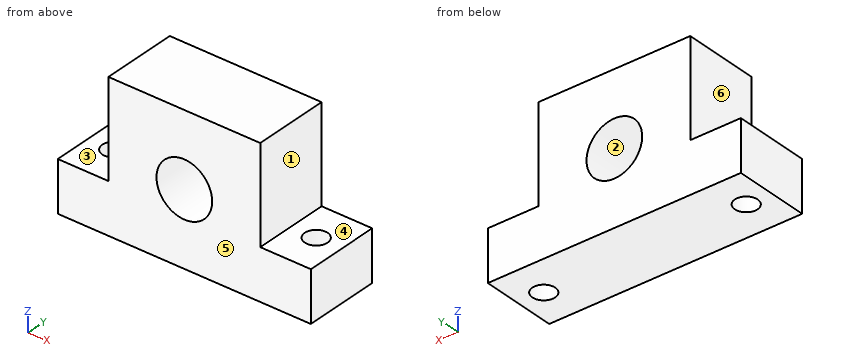
```python
from build123d import *

# Parameters (mm, degrees)
BOSS_EXTRUDE1_DEPTH  = 58
SKETCH3_R            = 11
CUT_EXTRUDE1_DEPTH   = 77.774006375
SKETCH4_W            = 20
SKETCH4_H            = 30
CUT_EXTRUDE2_DEPTH   = 38
M8_CLEARANCE_HOLE1_D = 9


with BuildPart() as part:
    # Sketch1 → Boss-Extrude1 (new body)
    with BuildSketch(Plane(origin=(0, 2.518676762, -29.699029015), x_dir=(1, 0, 0), z_dir=(0, 0, 1))):
        Polygon((-64.126560257, 671.967635092), (-14.126560257, 671.967635092), (35.873439743, 671.967635092), (35.873439743, 701.967635092), (-64.126560257, 701.967635092), align=None)
    extrude(amount=BOSS_EXTRUDE1_DEPTH)

    # Sketch3 → Cut-Extrude1 (cut, through all)
    with BuildSketch(Plane.XZ.offset(-674.486311854)):
        with Locations(Location((-14.126560257, -0.699029015, 0), (0, 0, 270))):
            Circle(SKETCH3_R)
    extrude(amount=-CUT_EXTRUDE1_DEPTH, mode=Mode.SUBTRACT)

    # Sketch4 → Cut-Extrude2 (cut)
    with BuildSketch(Plane.XY.offset(28.300970985)):
        with Locations((-54.126560257, 689.486311854)):
            Rectangle(SKETCH4_W, SKETCH4_H)
        with Locations((25.873439743, 689.486311854)):
            Rectangle(SKETCH4_W, SKETCH4_H)
    extrude(amount=-CUT_EXTRUDE2_DEPTH, mode=Mode.SUBTRACT)

    # M8 Clearance Hole1 (through all)
    with Locations(Plane(origin=(-5.422124321, 631.407959219, -9.699029015), x_dir=(1, 0, 0), z_dir=(0, 0, 1))):
        with Locations((-48.704435936, -458.836111538), (-48.704435936, -493.836111538), (31.295564064, -458.836111538), (31.295564064, -493.836111538), (-48.704435936, 58.078352635), (31.295564064, 58.078352635)):
            Hole(M8_CLEARANCE_HOLE1_D / 2)


solid = part.part
```
Geometry: final body of the model. Coordinates: model frame, mm. Face numbers are marked on the shaded views. A direction names the side the tool comes from. Coordinates: 2 decimals unless noted, no trailing zeros. Order: outer loops, then holes, each group sorted by start corner. A loop starts at its lowest first (then second) coordinate and runs counter-clockwise, first axis right, second up. Notation, with made-up numbers: M 45,62.25 L 90,62.25 A35 ccw 90,95.25 Z; hole C -28,68 d3. An arc over 180 degrees is marked long. Answer in a Markdown table with one row per item. Add a question column.
Q1. Reachability of the marked faces 4, 5 and 6 from +Z, -Z, +X, -X, +Y, -Y: full face, straight path, thin tool, end or side. Return the list, or none.
Q2. Section query B-B on x = 22.5. Return the cut outline in (y, z).
Q3. Section query C-C on y = 684. Return the cut outline in (x, z).
Q4. Section query A-A on z = -8. Return the cut outline in (x, y).
Q5. Line query: L1, parallel to Z at x = -14, y = 689; L2, parallel to Z at x = -45, y = 679.5; L3, parallel to X at y = 687, z = 2. Output: solid intervals per line, ascending.
Q6. Contact query for flat-ended pins moving along their axis: P1, Ø15, axis at y = 691, z = 10.5, coming from the -X side; P2, Ø16, axis at x = 30.5, y = 693.5, coming from the +Z side. Output: stop coordinate, or through.
Q7. Section query D-D on z = -16. Return the cut outline in (x, y).
Q8. Mould query, pull axis Z, two halves, no side actions, for the marked faces 1, 2 and 3. Classes: released by +Z, released by -Z, zero draft, split by the parting line, or undercut.
Completed:
| question | item | result |
|---|---|---|
| 1 | face 4 | +Z, +X, +Y, -Y |
| 1 | face 5 | +Z, -Z, +X, -X, -Y |
| 1 | face 6 | +Z, -X, +Y, -Y |
| 2 | outline | M 674.49,-29.7 L 686.51,-29.7 L 686.51,-9.7 L 674.49,-9.7 Z; M 692.46,-29.7 L 704.49,-29.7 L 704.49,-9.7 L 692.46,-9.7 Z |
| 3 | outline | M -64.13,-29.7 L 35.87,-29.7 L 35.87,-9.7 L 15.87,-9.7 L 15.87,28.3 L -44.13,28.3 L -44.13,-9.7 L -64.13,-9.7 Z; hole C -14.13,-0.7 d22 |
| 4 | outline | M -44.13,674.49 L -22.35,674.49 L -22.35,704.49 L -44.13,704.49 Z; M -5.9,674.49 L 15.87,674.49 L 15.87,704.49 L -5.9,704.49 Z |
| 5 | L1 | z = -29.7 to -11.7, 10.3 to 28.3 |
| 5 | L2 | z = -29.7 to -9.7 |
| 5 | L3 | x = -44.13 to -24.79, -3.46 to 15.87 |
| 6 | P1 | stops at x = -44.13 |
| 6 | P2 | stops at z = -9.7 |
| 7 | outline | M -64.13,674.49 L 35.87,674.49 L 35.87,704.49 L -64.13,704.49 Z; hole C -54.13,689.49 d9; hole C 25.87,689.49 d9 |
| 8 | face 1 | zero draft |
| 8 | face 2 | undercut |
| 8 | face 3 | released by +Z |
